from build123d import *

# Parameters (mm, degrees)
MAIN_BOARD_DEPTH    = 1.2
SKETCH2_R           = 0.9
DETAIL_CUTS_DEPTH   = 1.2
CHAMFER1_SIZE       = 0.25
SKETCH3_W           = 9
SKETCH3_H           = 11.5
SOC1_DEPTH          = 0.65
SOC1_DEPTH_BACK     = 1.85
SKETCH4_W           = 2
SKETCH4_H           = 3
SOC2_DEPTH          = 0.65
SKETCH5_W           = 35
SKETCH5_H           = 2.55
SKETCH5_W_2         = 28
CONTACTS_DEPTH      = 0.1
CONTACTS_DEPTH_BACK = 1.3


with BuildPart() as part:
    # Sketch1 → Main Board (new body)
    with BuildSketch(Plane.XY):
        Polygon((-34.2, 15), (-34.8, 14.4), (-34.8, -14.4), (-34.2, -15), (34.2, -15), (34.8, -14.4), (34.8, 14.4), (34.2, 15), align=None)
    extrude(amount=MAIN_BOARD_DEPTH)

    # Sketch2 → Detail Cuts (cut)
    with BuildSketch(Plane.XY.offset(1.2)):
        with Locations((-32.8, -9)):
            Circle(SKETCH2_R)
        with Locations((32.8, -9)):
            Circle(SKETCH2_R)
        with BuildLine():
            Line((-36.55, 3), (-33.7, 3))
            ThreePointArc((-33.7, 3), (-33.240380592, 3.190380592), (-33.05, 3.65))
            Line((-33.05, 3.65), (-33.05, 6.35))
            ThreePointArc((-33.05, 6.35), (-33.240380592, 6.809619408), (-33.7, 7))
            Line((-33.7, 7), (-36.55, 7))
            Line((-36.55, 7), (-36.55, 3))
        make_face()
        with BuildLine():
            Line((33.05, 3.65), (33.05, 6.35))
            ThreePointArc((33.05, 6.35), (33.240380592, 6.809619408), (33.7, 7))
            Line((33.7, 7), (36.55, 7))
            Line((36.55, 7), (36.55, 3))
            Line((36.55, 3), (33.7, 3))
            ThreePointArc((33.7, 3), (33.240380592, 3.190380592), (33.05, 3.65))
        make_face()
        with BuildLine():
            Line((3, -15), (3, -11.5))
            ThreePointArc((3, -11.5), (3.5, -11), (4, -11.5))
            Line((4, -11.5), (4, -15))
            ThreePointArc((4, -15), (3.5, -15.5), (3, -15))
        make_face()
    extrude(amount=-DETAIL_CUTS_DEPTH, mode=Mode.SUBTRACT)

    # Chamfer1
    chamfer1_edges = [part.edges().sort_by_distance(p)[0] for p in [
        (4, -15, 0.6),
        (3, -15, 0.6),
    ]]
    chamfer(chamfer1_edges, length=CHAMFER1_SIZE)

    # Sketch3 → SOC1 (add, two sides)
    with BuildSketch(Plane(origin=(0, 0, 0), x_dir=(-1, 0, 0), z_dir=(0, 0, -1))) as soc1_sk:
        with Locations((-20.8, 8.5)):
            Rectangle(SKETCH3_W, SKETCH3_H)
        with Locations((-9.3, 8.5)):
            Rectangle(SKETCH3_W, SKETCH3_H)
        with Locations((10.8, -3.5)):
            Rectangle(SKETCH3_W, SKETCH3_H)
        with Locations((-22.3, -3.5)):
            Rectangle(SKETCH3_W, SKETCH3_H)
        with Locations((-10.8, -3.5)):
            Rectangle(SKETCH3_W, SKETCH3_H)
        with Locations((22.3, -3.5)):
            Rectangle(SKETCH3_W, SKETCH3_H)
        with Locations((9.3, 8.5)):
            Rectangle(SKETCH3_W, SKETCH3_H)
        with Locations((20.8, 8.5)):
            Rectangle(SKETCH3_W, SKETCH3_H)
    extrude(amount=SOC1_DEPTH)
    extrude(soc1_sk.sketch, amount=-SOC1_DEPTH_BACK)

    # Sketch4 → SOC2 (add)
    with BuildSketch(Plane.XY.offset(1.2)):
        with Locations((0, 9.75)):
            Rectangle(SKETCH4_W, SKETCH4_H)
    extrude(amount=SOC2_DEPTH)

    # Sketch5 → Contacts (add, two sides)
    with BuildSketch(Plane.XY.offset(1.2)) as contacts_sk:
        with Locations((-15.25, -13.725)):
            Rectangle(SKETCH5_W, SKETCH5_H)
        with Locations((18.75, -13.725)):
            Rectangle(SKETCH5_W_2, SKETCH5_H)
    extrude(amount=CONTACTS_DEPTH)
    extrude(contacts_sk.sketch, amount=-CONTACTS_DEPTH_BACK)


solid = part.part
Here's how the part is built. I have some questions about the finished solid (model axes, mm). A direction names the side the tool comes from. Round coordinates to 2 decimals unless told otherwise and drop trailing zeros. Write each loop counter-clockwise with the first axis right and the second up, starting at its lowest first coordinate (ties: lowest second). Pieces come first, ordered by that corner, then holes.
1. For faces 5 (the flat face through (-11, -3, 1.85)), 6 (the flat face through (-15, -14, -0.1)), which set-ups out of +Z, -Z, +X, -X, +Y, -Y let a thin tool reach every point of the face, with its end or its side?
2. If we mould it in two halves opening along Y, with no side actions, what happens to faces 1 (the flat face through (0, 0, 0)), 2 (the flat face through (0, 15, 1)), 3 (the flat face through (19, -14, -0.1)), 4 (the cylindrical face through (-33.7, -9, 0.6))? For each: released by +Y, released by -Y, zero draft, split by the parting line, or undercut.
3. I need wall thicknesses on L1, parallel to X at y = -3.75, z = -0.25; L2, parallel to Y at x = 19, z = 1.25; L3, parallel to Y at x = 32.8, z = 0.4. Which ranges of each line are inside material? Lowest first, please.
4. Suppose I cut it at B-B (x = 0). List the corners of the cut face in (y, z) for me, and give its area (3 significant figures).
5. Will these pins go through, and if not, where does the flat tip stop? pin 1 Ø0.5 at (x, z) = (12, 1.5) entering from -Y; pin 2 Ø0.5 at (y, z) = (-6, 1.5) entering from +X; pin 3 Ø0.7 at (x, z) = (11, -0.5) entering from -Y; pin 4 Ø0.5 at (x, z) = (9.5, -0.5) entering from +Y.
6. Suppose I cut it at A-A (x = 22.5). List the corners of the cut face in (y, z) for me, and give its area (3 significant figures).
Answer sheet:
1. face 5: +Z, +X, -X, +Y, -Y
1. face 6: -Z, +X, -X, -Y
2. face 1: undercut
2. face 2: released by +Y
2. face 3: zero draft
2. face 4: undercut
3. L1: x = -26.8 to -17.8, -15.3 to -6.3, 6.3 to 15.3, 17.8 to 26.8
3. L2: y = -15 to -12.45, -9.25 to 2.25, 2.75 to 14.25
3. L3: y = -15 to -9.9, -8.1 to 15
4. outline: (-15, -0.1) - (-12.45, -0.1) - (-12.45, 0) - (15, 0) - (15, 1.2) - (11.25, 1.2) - (11.25, 1.85) - (8.25, 1.85) - (8.25, 1.2) - (-12.45, 1.2) - (-12.45, 1.3) - (-15, 1.3) - close
4. area: 38.5 mm2
5. pin 1: stops at y = -15
5. pin 2: stops at x = 26.8
5. pin 3: stops at y = -9.25
5. pin 4: stops at y = 14.25
6. outline: (-15, -0.1) - (-12.45, -0.1) - (-12.45, 0) - (-9.25, 0) - (-9.25, -0.65) - (2.25, -0.65) - (2.25, 0) - (2.75, 0) - (2.75, -0.65) - (14.25, -0.65) - (14.25, 0) - (15, 0) - (15, 1.2) - (14.25, 1.2) - (14.25, 1.85) - (2.75, 1.85) - (2.75, 1.2) - (2.25, 1.2) - (2.25, 1.85) - (-9.25, 1.85) - (-9.25, 1.2) - (-12.45, 1.2) - (-12.45, 1.3) - (-15, 1.3) - close
6. area: 66.4 mm2
